Verification items for this drawing (mm, ordinates from the low corner). A direction names the side the tool comes from. Give positions to 0.01 mm unless a question says otherwise; leave off trailing zeros. Order: outer loops, then holes, each group sorted by start corner. A loop starts at its lowest first (then second) coordinate and runs counter-clockwise, first axis right, second up.
(1) Mould release check, pull along X, two halves, no side actions. Record for the marked faces 3, 4 and 5: pulls with the +X half, pulls with the -X half, needs draft (parallel to the pull), parting line crosses it, or undercut.
(2) Sectioned sample at C-C on x = 444. Record the cut outline in (y, z) (1 decimal).
(3) Sectioned sample at A-A on z = 257. Record the cut outline in (x, y), plus the area to 3 significant figures.
(4) Sectioned sample at B-B on y = 743. Record the cut outline in (x, z), plus the area to 3 significant figures.
(5) Sectioned sample at D-D on z = 527.5. Record the cut outline in (x, y).
(6) Scan lines: L1, parallel to Y at x = 508, z = 306; L2, parallel to Y at x = 250.5, z = 669; L3, parallel to Z at x = 925.5, y = 515.5. Record each from-to range of solid material in increasing order.
(7) Gauge pin test, flat end, axial feed: pin 1 (1.5 mm diameter, centred on x = 530, z = 433, fed in from +Y) (1 decimal). Record the tip position at first contact, or that the pin passes through.
(8) Access from +Z, -Z, +X, -X, +Y, -Y to the whole of each face (thin tool, end or side, straight path). Record for the marked faces 1 and 2.
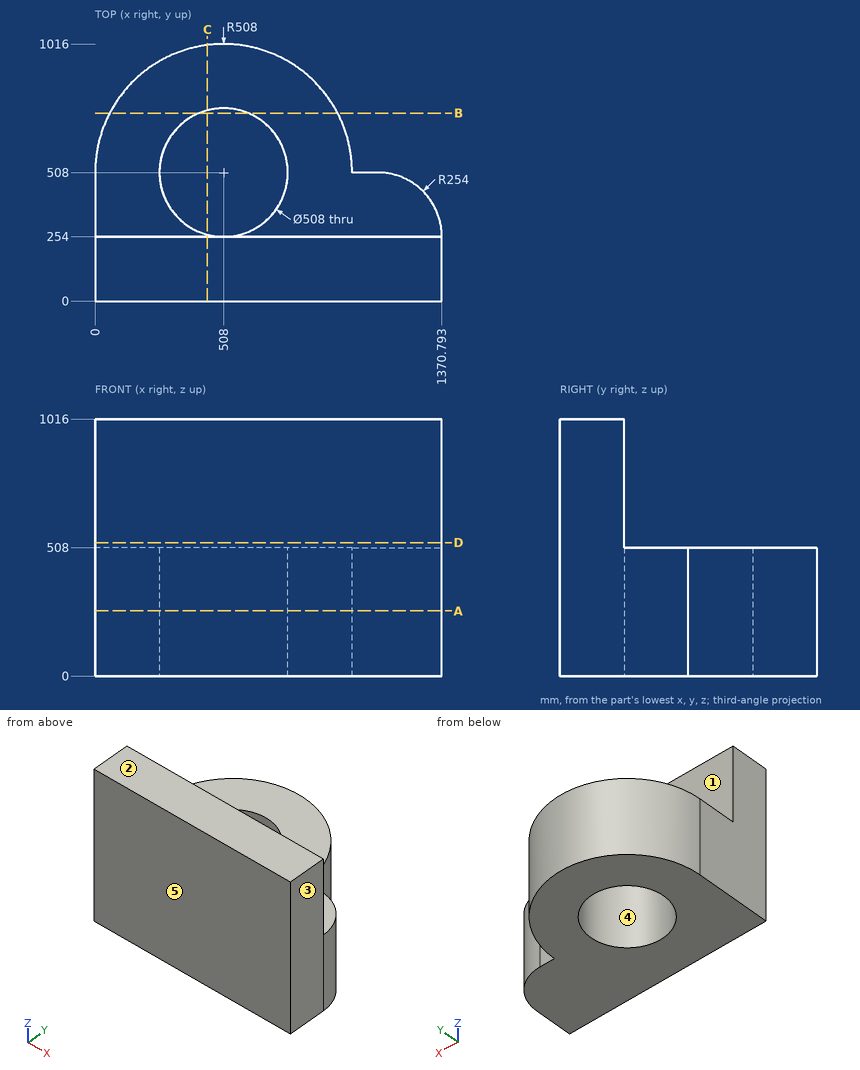
Ans:
1. face 3: pulls with the +X half
1. face 4: undercut
1. face 5: needs draft
2. outline: (0, 0) - (262.2, 0) - (262.2, 508) - (254, 508) - (254, 1016) - (0, 1016) - close; (753.8, 0) - (1012, 0) - (1012, 508) - (753.8, 508) - close
3. outline: (0, 0) - (1370.79, 0) - (1370.79, 254) arc R254 ccw to (1116.79, 508) - (1016, 508) arc R508 ccw to (0, 508) - close; hole circle Ø508 at (508, 508)
3. area: 885,000 mm2
4. outline: (57.62, 0) - (411.61, 0) - (411.61, 508) - (57.62, 508) - close; (604.39, 0) - (958.38, 0) - (958.38, 508) - (604.39, 508) - close
4. area: 360,000 mm2
5. outline: (0, 0) - (1370.79, 0) - (1370.79, 254) - (0, 254) - close
6. L1: y = 0 to 254, 762 to 1016
6. L2: y = 0 to 254
6. L3: z = 0 to 508
7. pin 1: stops at y = 1015.6
8. face 1: +Z, +X, -X, +Y
8. face 2: +Z, +X, -X, +Y, -Y
